```python
from build123d import *

# Parameters (mm, degrees)
SKETCH1_W           = 55
SKETCH1_H           = 30.75
BOSS_EXTRUDE1_DEPTH = 50
CUT_EXTRUDE1_DEPTH  = 50
CUT_EXTRUDE2_DEPTH  = 81.439806688
BOSS_EXTRUDE2_REACH = 82.44
SKETCH6_R           = 13.75
CUT_EXTRUDE3_DEPTH  = 81.212608111
CUT_EXTRUDE4_DEPTH  = 81.439806688
SKETCH8_R           = 6
CUT_EXTRUDE5_DEPTH  = 72.014963212
CUT_EXTRUDE6_DEPTH  = 72.014963212
SKETCH10_W          = 55
SKETCH10_H          = 4.5
CUT_EXTRUDE7_DEPTH  = 70.055231518
FILLET5_R           = 1
FILLET6_R           = 5
CUT_EXTRUDE8_DEPTH  = 68.172352944
SKETCH17_W          = 55
SKETCH17_H          = 6
BOSS_EXTRUDE4_DEPTH = 22
BOSS_EXTRUDE5_DEPTH = 55
SKETCH19_W          = 55
SKETCH19_H          = 16.3
CUT_EXTRUDE9_DEPTH  = 0.75
BOSS_EXTRUDE6_DEPTH = 55


with BuildPart() as part:
    # Sketch1 → Boss-Extrude1 (new body)
    with BuildSketch(Plane(origin=(0, 0, 0), x_dir=(1, 0, 0), z_dir=(0, 1, 0))):
        with Locations((27.5, 15.375)):
            Rectangle(SKETCH1_W, SKETCH1_H)
    extrude(amount=BOSS_EXTRUDE1_DEPTH)

    # Sketch4 → Cut-Extrude1 (cut)
    with BuildSketch(Plane(origin=(55, 0, 0), x_dir=(0, 0, -1), z_dir=(1, 0, 0))):
        Polygon((-27.355339059, 45.355339059), (8, 80.710678119), (43.355339059, 45.355339059), (8, 10), align=None)
    extrude(amount=-CUT_EXTRUDE1_DEPTH, mode=Mode.SUBTRACT)

    # Sketch5 → Cut-Extrude2 (cut, through all)
    with BuildSketch(Plane(origin=(55, 0, 0), x_dir=(0, 0, -1), z_dir=(1, 0, 0))):
        Polygon((-11.642135624, 15.5), (-4.571067812, 22.571067812), (2.5, 15.5), (-4.571067812, 8.428932188), align=None)
    extrude(amount=-CUT_EXTRUDE2_DEPTH, mode=Mode.SUBTRACT)

    # Sketch12 → Boss-Extrude2 (add, up to next)
    with BuildSketch(Plane(origin=(55, 0, 0), x_dir=(0, 0, -1), z_dir=(1, 0, 0)), mode=Mode.PRIVATE) as boss_extrude2_sk1:
        Polygon((2.5, 15.5), (8, 10), (8.707106781, 10.707106781), (3.207106781, 16.207106781), align=None)
    boss_extrude2_tool1 = extrude(boss_extrude2_sk1.sketch, amount=-BOSS_EXTRUDE2_REACH, mode=Mode.PRIVATE) - part.part
    add(boss_extrude2_tool1.solids().sort_by_distance((55, 13.103553, -5.603553))[0])

    # Sketch6 → Cut-Extrude3 (cut, through all)
    with BuildSketch(Plane(origin=(0, 1, 1), x_dir=(1, 0, 0), z_dir=(0, 0.7071067811865515, 0.7071067811865436))):
        with Locations((12, 23.692388155)):
            Circle(SKETCH6_R)
    extrude(amount=CUT_EXTRUDE3_DEPTH, mode=Mode.SUBTRACT)

    # Sketch7 → Cut-Extrude4 (cut, through all)
    with BuildSketch(Plane(origin=(55, 0, 0), x_dir=(0, 0, -1), z_dir=(1, 0, 0))):
        Polygon((0, 13), (5.506338941, 18.506338941), (11.006338941, 13.006338941), (61, 63), (25.408423261, 63), (0, 63), align=None)
    extrude(amount=-CUT_EXTRUDE4_DEPTH, mode=Mode.SUBTRACT)

    # Sketch8 → Cut-Extrude5 (cut, through all)
    with BuildSketch(Plane(origin=(0, 0, 0), x_dir=(1, 0, 0), z_dir=(0, 1, 0))):
        with Locations((25.75, 32.25)):
            Circle(SKETCH8_R)
    extrude(amount=CUT_EXTRUDE5_DEPTH, mode=Mode.SUBTRACT)

    # Sketch9 → Cut-Extrude6 (cut, through all)
    with BuildSketch(Plane(origin=(55, 0, 0), x_dir=(0, 0, -1), z_dir=(1, 0, 0))):
        Polygon((26.25, 28.25), (30.75, 28.25), (30.75, 32.75), align=None)
    extrude(amount=-CUT_EXTRUDE6_DEPTH, mode=Mode.SUBTRACT)

    # Sketch10 → Cut-Extrude7 (cut, through all)
    with BuildSketch(Plane(origin=(0, 0, 0), x_dir=(1, 0, 0), z_dir=(0, 1, 0))):
        with Locations((27.5, 28.5)):
            Rectangle(SKETCH10_W, SKETCH10_H)
    extrude(amount=CUT_EXTRUDE7_DEPTH, mode=Mode.SUBTRACT)

    # Fillet5
    fillet5_edges = [part.edges().sort_by_distance(p)[0] for p in [
        (0, 15.756338941, -8.256338941),
    ]]
    fillet(fillet5_edges, radius=FILLET5_R)

    # Fillet6
    fillet6_edges = [part.edges().sort_by_distance(p)[0] for p in [
        (21.474804244, 13.457106781, -5.957106781),
    ]]
    fillet(fillet6_edges, radius=FILLET6_R)

    # Sketch16 → Cut-Extrude8 (cut, through all)
    with BuildSketch(Plane(origin=(55, 0, 0), x_dir=(0, 0, -1), z_dir=(1, 0, 0))):
        Polygon((26.25, 20.75), (9.25, 3.75), (0, 13), (0, 0), (26.25, 0), align=None)
    extrude(amount=-CUT_EXTRUDE8_DEPTH, mode=Mode.SUBTRACT)

    # Sketch17 → Boss-Extrude4 (add)
    with BuildSketch(Plane(origin=(0, 0, -26.25), x_dir=(-1, 0, 0), z_dir=(0, 0, -1))):
        with Locations((-27.5, 25.25)):
            Rectangle(SKETCH17_W, SKETCH17_H)
    extrude(amount=BOSS_EXTRUDE4_DEPTH)

    # Sketch18 → Boss-Extrude5 (add)
    with BuildSketch(Plane(origin=(55, 0, 0), x_dir=(0, 0, -1), z_dir=(1, 0, 0))):
        Polygon((17.75, 12.25), (33.75, 28.25), (26.25, 28.25), (14, 16), align=None)
    extrude(amount=-BOSS_EXTRUDE5_DEPTH)

    # Sketch19 → Cut-Extrude9 (cut)
    with BuildSketch(Plane(origin=(0, 28.25, 0), x_dir=(1, 0, 0), z_dir=(0, 1, 0))):
        with Locations((27.5, 37.25)):
            Rectangle(SKETCH19_W, SKETCH19_H)
    extrude(amount=-CUT_EXTRUDE9_DEPTH, mode=Mode.SUBTRACT)

    # Sketch20 → Boss-Extrude6 (add)
    with BuildSketch(Plane(origin=(55, 0, 0), x_dir=(0, 0, -1), z_dir=(1, 0, 0))):
        Polygon((0, 13), (-1.060660172, 11.939339828), (8.189339828, 2.689339828), (9.25, 3.75), align=None)
    extrude(amount=-BOSS_EXTRUDE6_DEPTH)


solid = part.part
```
Check sheet for the modelled part. Datum: model origin and axes. Units: mm. A direction names the side the tool comes from. Round coordinates to 2 decimals unless told otherwise and drop trailing zeros. Write each loop counter-clockwise with the first axis right and the second up, starting at its lowest first coordinate (ties: lowest second). Pieces come first, ordered by that corner, then holes. Notation, with made-up numbers: M -25,29.25 L 11,29.25 A13 cw 11,46.25 Z; hole C 50,85 d10. An arc over 180 degrees is marked long. Write item = value, one per line. Start each with the question number.
1. Section check A-A, the plane x = 34. Record the cut outline in (y, z), then the cut area to 3 significant figures.
2. Tool access check on faces 4 (the flat face through (27, 27.5, -37)), 5 (the flat face through (39.371, 13.419, -5.996)), 6 (the flat face through (27.88, 7.38, -3.5)), 7 (the flat face through (28, 22.25, -38)). Record the directions out of +Z, -Z, +X, -X, +Y, -Y that give a thin tool (end or side, any length) a straight path to the whole face; none if there is none.
3. Release check for a two-part mould opening along X. For faces 1 (the flat face through (0, 17, -22)), 2 (the flat face through (28, 28.25, -28)), 3 (the flat face through (55, 17, -22)) record: pulls with the +X half, pulls with the -X half, needs draft (parallel to the pull), parting line crosses it, or undercut.
4. Section check C-C, the plane y = 6.25. Record the cut outline in (x, z), then the cut area to 3 significant figures.
5. Scan lines: line 1 (Z direction, x = 31, y = 15); line 2 (Y direction, x = 4.5, z = -38); line 3 (Z direction, x = 4, y = 7.25). Record each from-to range of solid material in increasing order. Write a range as [from, to].
6. Gauge pin test, flat ends, axial feed: pin 1 (1 mm diameter, centred on y = 10, z = -8.5, fed in from -X); pin 2 (6 mm diameter, centred on x = 26, y = 6.5, fed in from +Z); pin 3 (4 mm diameter, centred on x = 28, z = -40, fed in from +Y); pin 4 (1 mm diameter, centred on y = 14, z = -7.5, fed in from -X). Record the tip position at first contact, or that the pin passes through.
7. Section check B-B, the plane z = -31. Record the cut outline in (x, y).
8. Section check D-D, the plane x = 18. Record the cut outline in (y, z).
Results found:
q1.outline = M 2.69,-8.19 L 22.25,-27.75 L 22.25,-48.25 L 28.25,-48.25 L 28.25,-45.4 L 27.5,-45.4 L 27.5,-29.1 L 28.25,-29.1 L 28.25,-26.25 L 10.71,-8.71 L 16.21,-3.21 L 11.94,1.06 Z
q1.area = 317 mm^2
q2.face_4 = +X, -X, +Y
q2.face_5 = +X, +Y
q2.face_6 = +Z, +X, -X, -Y
q2.face_7 = -Z, +X, -X, -Y
q3.face_1 = pulls with the -X half
q3.face_2 = needs draft
q3.face_3 = pulls with the +X half
q4.outline = M 0,-11.75 L 55,-11.75 L 55,-4.63 L 0,-4.63 Z
q4.area = 392 mm^2
q5.line_1 = [-20.5, -13], [-4.41, -2]
q5.line_2 = [22.25, 27.5]
q5.line_3 = [-12.75, -3.63]
q6.pin_1 = 0
q6.pin_2 = -1.38
q6.pin_3 = 27.5
q6.pin_4 = 0.45
q7.outline = M 0,22.25 L 55,22.25 L 55,27.5 L 0,27.5 Z
q8.outline = M 2.69,-8.19 L 22.25,-27.75 L 22.25,-48.25 L 28.25,-48.25 L 28.25,-45.4 L 27.5,-45.4 L 27.5,-29.1 L 28.25,-29.1 L 28.25,-26.25 L 9,-7 L 14.5,-1.5 L 11.94,1.06 Z
